```python
from build123d import *

# Parameters (mm, degrees)
SKETCH1_W                = 99.5
SKETCH1_H                = 66
BOSS_EXTRUDE1_DEPTH      = 3.175
CUT_EXTRUDE1_DEPTH       = 60.784137737
M3_CLEARANCE_HOLE1_D     = 3.2
M3_CLEARANCE_HOLE1_DEPTH = 12
M3_CLEARANCE_HOLE1_TIP   = 0.96137699
SKETCH6_W                = 3.175
SKETCH6_H                = 8
SKETCH6_W_2              = 8
SKETCH6_H_2              = 3.175
BOSS_EXTRUDE2_DEPTH      = 3.175
FILLET1_R                = 3
FILLET2_R                = 1


with BuildPart() as part:
    # Sketch1 → Boss-Extrude1 (new body)
    with BuildSketch(Plane.XY):
        Rectangle(SKETCH1_W, SKETCH1_H)
    extrude(amount=BOSS_EXTRUDE1_DEPTH)

    # Sketch2 → Cut-Extrude1 (cut, through all)
    with BuildSketch(Plane.XY.offset(3.175)):
        Polygon((-42.75, 24.756797808), (-5.427251789, 0), (-42.75, -24.756797808), align=None)
        Polygon((33.769717908, 26), (0, 3.599986111), (-33.769717908, 26), align=None)
        Polygon((42.75, 24.756797808), (5.427251789, 0), (42.75, -24.756797808), align=None)
        Polygon((-33.769717908, -26), (33.769717908, -26), (0, -3.599986111), align=None)
    extrude(amount=-CUT_EXTRUDE1_DEPTH, mode=Mode.SUBTRACT)

    # M3 Clearance Hole1
    with Locations(Plane.XY.offset(3.175)):
        with Locations((0, -29.5)):
            Hole(M3_CLEARANCE_HOLE1_D / 2, depth=M3_CLEARANCE_HOLE1_DEPTH)
            with Locations((0, 0, -(M3_CLEARANCE_HOLE1_DEPTH + M3_CLEARANCE_HOLE1_TIP / 2))):  # 118° drill point
                Cone(0, M3_CLEARANCE_HOLE1_D / 2, M3_CLEARANCE_HOLE1_TIP, mode=Mode.SUBTRACT)

    # Sketch6 → Boss-Extrude2 (add)
    with BuildSketch(Plane.XY.offset(3.175)):
        with Locations((-51.3375, 15)):
            Rectangle(SKETCH6_W, SKETCH6_H)
        with Locations((-51.3375, -15)):
            Rectangle(SKETCH6_W, SKETCH6_H)
        with Locations((-35, 34.5875)):
            Rectangle(SKETCH6_W_2, SKETCH6_H_2)
        with Locations((35, 34.5875)):
            Rectangle(SKETCH6_W_2, SKETCH6_H_2)
    extrude(amount=-BOSS_EXTRUDE2_DEPTH)

    # Fillet1
    fillet1_edges = [part.edges().sort_by_distance(p)[0] for p in [
        (42.75, 24.756797808, 1.5875),
        (42.75, -24.756797808, 1.5875),
        (5.427251789, 0, 1.5875),
        (-33.769717908, 26, 1.5875),
        (33.769717908, 26, 1.5875),
        (0, 3.599986111, 1.5875),
        (0, -3.599986111, 1.5875),
        (33.769717908, -26, 1.5875),
        (-33.769717908, -26, 1.5875),
        (-42.75, -24.756797808, 1.5875),
        (-42.75, 24.756797808, 1.5875),
        (-5.427251789, 0, 1.5875),
    ]]
    fillet(fillet1_edges, radius=FILLET1_R)

    # Fillet2
    fillet2_edges = [part.edges().sort_by_distance(p)[0] for p in [
        (49.75, -33, 1.5875),
        (-49.75, -33, 1.5875),
        (-49.75, 33, 1.5875),
        (49.75, 33, 1.5875),
    ]]
    fillet(fillet2_edges, radius=FILLET2_R)


solid = part.part
```
Geometry check sheet. Reference: the model listing, model coordinates, mm. A direction names the side the tool comes from. Coordinates: 2 decimals unless noted, no trailing zeros. Loops run counter-clockwise (first coordinate to the right, second up) from the corner with the lowest first, then second, coordinate; pieces in that order, holes last.
Item 1: Thickness scan on line 1 (Y direction, x = 0, z = 1.1); line 2 (Y direction, x = 10.5, z = 2.95); line 3 (X direction, y = 25.5, z = 2.5). Record the ranges inside material, lowest first.
Item 2: Sectioned sample at A-A, the plane x = 0. Record the boundary of the cut face in (y, z) (3 decimals).
Item 3: Sectioned sample at D-D, the plane z = 1. Count the separate pieces of the cut face and the enclosed holes in it, then the cut area to 3 significant figures.
Item 4: Go/stop test with flat-tipped pins: pin 1 Ø1 at (y, z) = (34, 2) entering from +X; pin 2 Ø1 at (y, z) = (35, 2) entering from -X; pin 3 Ø1 at (x, z) = (-51, 2) entering from -Y. Record where each tip stops, or that it passes through.
Item 5: Sectioned sample at C-C, the plane y = 18. Record the boundary of the cut face in (x, z) (3 decimals), then the cut area to 3 significant figures.
Item 6: Access from +Z, -Z, +X, -X, +Y, -Y to the whole of each face (thin tool, end or side, straight path). Record for faces 5 (the face through (-39, 35, 2)), 6 (the face through (-23.85, 12.22, 1.61)), 7 (the face through (-49.75, 0, 2)), 8 (the face through (44, 33, 2)).
Item 7: Release check for a two-part mould opening along Y. For faces 1 (the face through (-52.925, 15, 2)), 2 (the face through (0, 33, 2)), 3 (the face through (-51, -19, 2)), 4 (the face through (0, 26, 2)) record: released by +Y, released by -Y, zero draft, split by the parting line, or undercut.
Item 8: Sectioned sample at B-B, the plane y = -29.5. Record the boundary of the cut face in (x, z) (3 decimals).
Check result:
1. line 1: y = -33 to -31.1, -27.9 to -26, -4.2 to 4.2, 26 to 33
1. line 2: y = -33 to -26, -10.56 to -3.36, 3.36 to 10.56, 26 to 33
1. line 3: x = -49.75 to -25.48, 25.48 to 49.75
2. outline: (-33, 0) - (-31.1, 0) - (-31.1, 3.175) - (-33, 3.175) - close; (-27.9, 0) - (-26, 0) - (-26, 3.175) - (-27.9, 3.175) - close; (-4.2, 0) - (4.2, 0) - (4.2, 3.175) - (-4.2, 3.175) - close; (26, 0) - (33, 0) - (33, 3.175) - (26, 3.175) - close
3. separate pieces: 1
3. enclosed holes: 5
3. area: 3,410 mm2
4. pin 1: stops at x = 39
4. pin 2: stops at x = -39
4. pin 3: stops at y = -19
5. outline: (-52.925, 0) - (-42.75, 0) - (-42.75, 3.175) - (-52.925, 3.175) - close; (-32.564, 0) - (-21.709, 0) - (-21.709, 3.175) - (-32.564, 3.175) - close; (21.709, 0) - (32.564, 0) - (32.564, 3.175) - (21.709, 3.175) - close; (42.75, 0) - (49.75, 0) - (49.75, 3.175) - (42.75, 3.175) - close
5. area: 123 mm2
6. face 5: +Z, -Z, -X, +Y
6. face 6: +Z, -Z
6. face 7: +Z, -Z, -X
6. face 8: +Z, -Z, +X, +Y
7. face 1: zero draft
7. face 2: released by +Y
7. face 3: released by -Y
7. face 4: undercut
8. outline: (-49.75, 0) - (-1.6, 0) - (-1.6, 3.175) - (-49.75, 3.175) - close; (1.6, 0) - (49.75, 0) - (49.75, 3.175) - (1.6, 3.175) - close
